For this review, take the finished solid that the model builds, in its own axes (mm). Face numbers are marked on the shaded views. A direction names the side the tool comes from. Round coordinates to 2 decimals unless told otherwise and drop trailing zeros. Write each loop counter-clockwise with the first axis right and the second up, starting at its lowest first coordinate (ties: lowest second). Pieces come first, ordered by that corner, then holes. Notation, with made-up numbers: (-39, 62) -> (12, 62) arc R22 ccw to (12, 76) -> close; hole circle Ø4 at (5.25, 42). An arc over 180 degrees is marked (long way). Write each question's results on one line, items separated by ' | '. Start each with the question number.
Item 1: To check wall thickness, follow line 1 along X through (y, z) = (0.9, 2.5); line 2 along X through (y, z) = (1.25, -10); line 3 along Z through (x, y) = (2, 1.1). State the ranges of each line that lie inside material, in increasing order.
Item 2: Clearance check with flat-ended pins moving along their axes: pin 1 (1.5 mm diameter, centred on x = 20, y = 2, fed in from +Z); pin 2 (1 mm diameter, centred on x = 17.5, y = 1.5, fed in from -Z). State where each tip first meets the part, or that it passes through.
Item 3: Tool access review of the marked faces 1 and 2: name each direction out of +Z, -Z, +X, -X, +Y, -Y from which nothing blocks a thin tool from reaching the whole face with its end or side.
Item 4: The part is to be moulded in two halves that separate along X. For the marked faces 3, 4 and 5, say which applies: +X half, -X half, draft (parallel to the pull), parting line (faces both ways), or undercut.
Item 5: Add section B-B (x = 3.5). State the section outline as (y, z) points, plus the area to 3 significant figures.
Item 6: Add section C-C (y = 2.55). Count the separate pieces of the cut face and the enclosed holes in it, plus the area to 3 significant figures.
Item 7: Add section A-A (z = -10). State the section outline as (x, y) points, plus the area to 3 significant figures.
Item 8: Add section D-D (x = 21). State the section outline as (y, z) points.
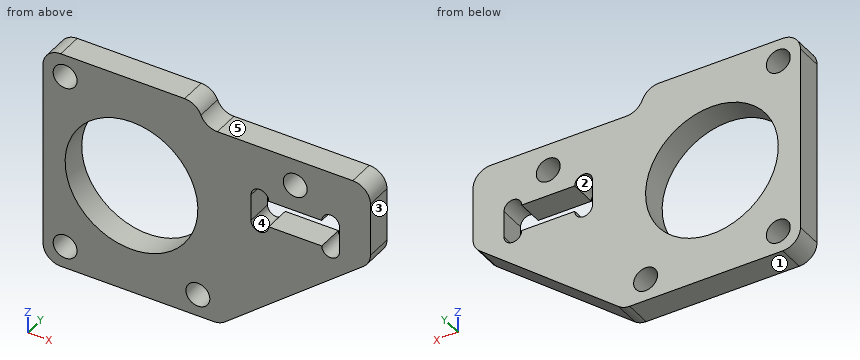
from build123d import *

# Parameters (mm, degrees)
SKETCH_1_R          = 7.5
EXTRUDE_1_DEPTH     = 3
SKETCH_3_R          = 1.35
CUT_EXTRUDE_1_DEPTH = 30.904013109
EXTRUDE_2_DEPTH     = 3
CUT_EXTRUDE_3_DEPTH = 30.904013109
FILLET_1_R          = 2
FILLET_2_R          = 2


with BuildPart() as part:
    # 草图1 → 凸台-拉伸1 (new body)
    with BuildSketch(Plane(origin=(0, 0, 0), x_dir=(1, 0, 0), z_dir=(0, 1, 0))):
        Polygon((-10, -12.5), (0, -12.5), (8, -12.5), (8, -10), (27, -10), (27, -4), (10, -4), (10, 12.5), (-10, 12.5), align=None)
        with Locations(Location((0, 0, 0), (0, 0, 270))):
            Circle(SKETCH_1_R, mode=Mode.SUBTRACT)
    extrude(amount=EXTRUDE_1_DEPTH)

    # 草图3 → 切除-拉伸1 (cut, through all)
    with BuildSketch(Plane(origin=(0, 3, 0), x_dir=(1, 0, 0), z_dir=(0, 1, 0))):
        with Locations(Location((18.5, -7, 0), (0, 0, 270))):
            Circle(SKETCH_3_R)
        with Locations(Location((-7.5, 10, 0), (0, 0, 270))):
            Circle(SKETCH_3_R)
        with Locations(Location((-7.5, -10, 0), (0, 0, 90))):
            Circle(SKETCH_3_R)
        with Locations(Location((7.5, 10, 0), (0, 0, 90))):
            Circle(SKETCH_3_R)
    extrude(amount=-CUT_EXTRUDE_1_DEPTH, mode=Mode.SUBTRACT)

    # 草图5 → 凸台-拉伸2 (add)
    with BuildSketch(Plane(origin=(0, 3, 0), x_dir=(1, 0, 0), z_dir=(0, 1, 0))):
        Polygon((23.5, -4), (27, -4), (27, -1), (10, 12.5), (10, -4), (13.5, -4), (13.5, -1), (23.5, -1), align=None)
    extrude(amount=-EXTRUDE_2_DEPTH)

    # 草图7 → 切除-拉伸3 (cut, through all)
    with BuildSketch(Plane(origin=(0, 3, 0), x_dir=(1, 0, 0), z_dir=(0, 1, 0))):
        with BuildLine():
            Line((23.5, -1), (21.5, -1))
            ThreePointArc((21.5, -1), (22.5, 0), (23.5, -1))
        make_face()
        with BuildLine():
            Line((13.5, -1), (15.5, -1))
            ThreePointArc((15.5, -1), (14.5, 0), (13.5, -1))
        make_face()
        with BuildLine():
            Line((13.5, -4), (15.5, -4))
            ThreePointArc((15.5, -4), (14.5, -5), (13.5, -4))
        make_face()
        with BuildLine():
            Line((23.5, -4), (21.5, -4))
            ThreePointArc((21.5, -4), (22.5, -5), (23.5, -4))
        make_face()
    extrude(amount=-CUT_EXTRUDE_3_DEPTH, mode=Mode.SUBTRACT)

    # 圆角1
    fillet_1_edges = [part.edges().sort_by_distance(p)[0] for p in [
        (27, 1.5, 10),
        (8, 1.5, 12.5),
        (-10, 1.5, 12.5),
        (-10, 1.5, -12.5),
    ]]
    fillet(fillet_1_edges, radius=FILLET_1_R)

    # 圆角2
    fillet_2_edges = [part.edges().sort_by_distance(p)[0] for p in [
        (8, 1.5, 10),
        (10, 1.5, -12.5),
        (27, 1.5, 1),
    ]]
    fillet(fillet_2_edges, radius=FILLET_2_R)


solid = part.part
Responses:
1) line 1: x = -10 to -7.07, 7.07 to 13.5, 23.5 to 27 | line 2: x = -10 to -8.85, -6.15 to 6.15, 8.85 to 13.15 | line 3: z = -12.5 to -7.23, 7.23 to 12.5
2) pin 1: stops at z = 10 | pin 2: stops at z = -6.94
3) face 1: -Z, +X, -X, +Y, -Y | face 2: +Y, -Y
4) face 3: +X half | face 4: undercut | face 5: draft
5) outline: (0, -12.5) -> (3, -12.5) -> (3, -6.63) -> (0, -6.63) -> close; (0, 6.63) -> (3, 6.63) -> (3, 12.5) -> (0, 12.5) -> close | area: 35.2 mm^2
6) separate pieces: 1 | enclosed holes: 6 | area: 524 mm^2
7) outline: (-10, 0) -> (-8.85, 0) -> (-8.85, 3) -> (-10, 3) -> close; (-6.15, 0) -> (6.15, 0) -> (6.15, 3) -> (-6.15, 3) -> close; (8.85, 0) -> (13.15, 0) -> (13.15, 3) -> (8.85, 3) -> close | area: 53.2 mm^2
8) outline: (0, -3.76) -> (3, -3.76) -> (3, 1) -> (0, 1) -> close; (0, 4) -> (3, 4) -> (3, 10) -> (0, 10) -> close
